Can you work these out from the drawing? Everything is in mm from the part's minimum corner. Coordinates: 2 decimals unless noted, no trailing zeros. Order: outer loops, then holes, each group sorted by start corner. A loop starts at its lowest first (then second) coordinate and runs counter-clockwise, first axis right, second up. Notation, with made-up numbers: (45.25, 44) - (73.25, 44) arc R29 ccw to (73.25, 75) - close; hole circle Ø4 at (25, -2.5). An arc over 180 degrees is marked (long way). Use a Markdown table: item, result. Add a question column.
(1) I want a section at B-B (x = 12.5). List the corners of the cut face in (y, z) for me, and give its area (3 significant figures).
(2) I want a section at C-C (y = 93). List the corners of the cut face in (x, z) for me.
(3) I want a section at A-A (z = 12.5). List the corners of the cut face in (x, y) for me.
(4) If I drill on L1, parallel to X at y = 78, z = 12.5; L2, parallel to X at y = 31, z = 13.25, over which ranges is the centre line in solid material (lowest first)? Write a range as [from, to].
(5) For pin 1 Ø2 at (y, z) = (12, 21) entering from -X; pin 2 Ø1 at (y, z) = (68, 5.5) entering from +X; pin 3 Ø5 at (y, z) = (65.5, 6) entering from +X; pin 4 Ø6.5 at (x, z) = (12.5, 12.5) entering from -Y, each with a flat end and sliding along its axis, tell me the tip position at first contact or that it passes through.
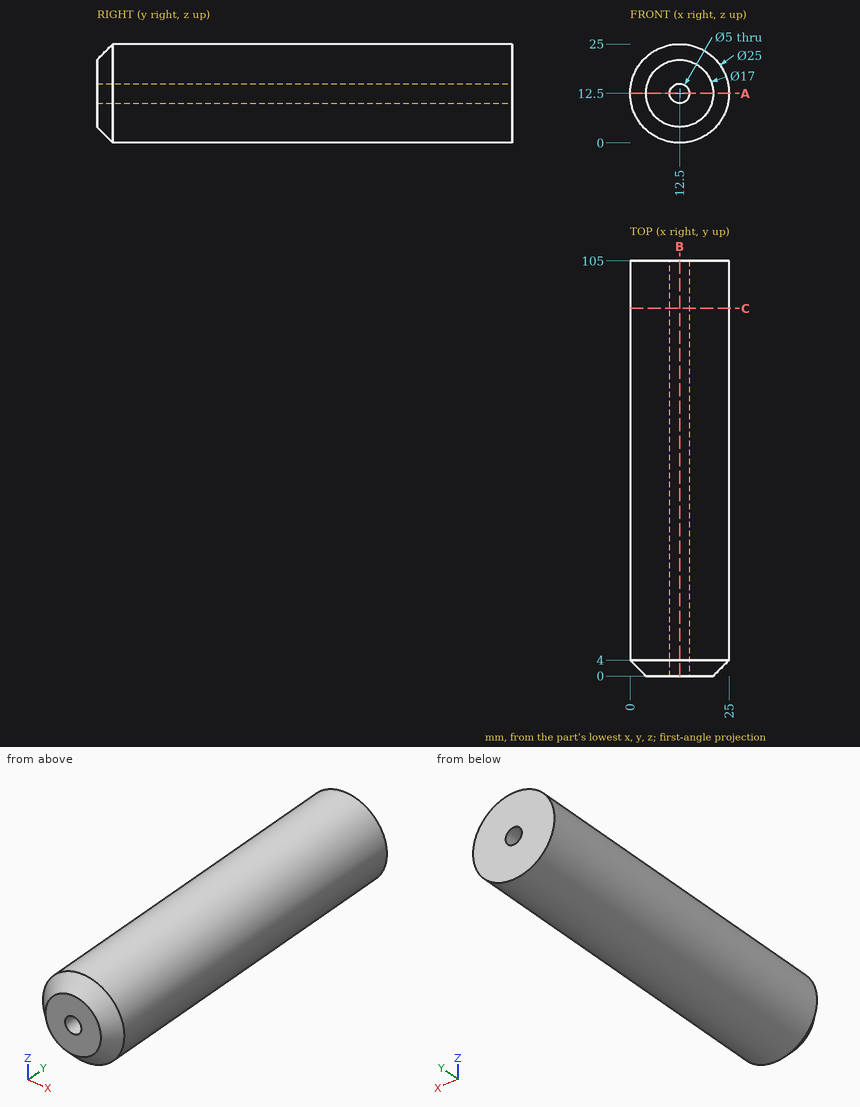
Answers follow:
| question | item | result |
|---|---|---|
| 1 | outline | (0, 4) - (4, 0) - (105, 0) - (105, 10) - (0, 10) - close; (0, 15) - (105, 15) - (105, 25) - (4, 25) - (0, 21) - close |
| 1 | area | 2,080 mm² |
| 2 | outline | circle Ø25 at (12.5, 12.5); hole circle Ø5 at (12.5, 12.5) |
| 3 | outline | (0, 4) - (4, 0) - (10, 0) - (10, 105) - (0, 105) - close; (15, 0) - (21, 0) - (25, 4) - (25, 105) - (15, 105) - close |
| 4 | L1 | x = [0, 10], [15, 25] |
| 4 | L2 | x = [0.02, 10.12], [14.88, 24.98] |
| 5 | pin 1 | stops at x = 2.5 |
| 5 | pin 2 | stops at x = 23.18 |
| 5 | pin 3 | stops at x = 24.34 |
| 5 | pin 4 | stops at y = 0 |
